```python
from build123d import *

# Parameters (mm, degrees)
F0_W     = 60
F0_H     = 40
F1_DEPTH = 10
F2_W     = 20
F2_H     = 40
F3_DEPTH = 20
F4_W     = 20
F4_H     = 10.2027570456
F5_DEPTH = 10
F6_DEPTH = 10


with BuildPart() as f1:
    # F0 (on Top) → F1 (new body)
    with BuildSketch(Plane.XY):
        with Locations((30, 20)):
            Rectangle(F0_W, F0_H)
    extrude(amount=F1_DEPTH)

    # F2 (on face) → F3 (join)
    with BuildSketch(Plane.XY.offset(10)):
        with Locations((10, 20)):
            Rectangle(F2_W, F2_H)
    extrude(amount=F3_DEPTH)

    # F4 (on face) → F5 (join)
    with BuildSketch(Plane.XY.offset(10)):
        with Locations((30, 34.8986214772)):
            Rectangle(F4_W, F4_H)
        with Locations((30, 5.1013785228)):
            Rectangle(F4_W, F4_H)
    extrude(amount=F5_DEPTH)

    # F4 (on face) → F6 (join)
    with BuildSketch(Plane.XY.offset(10)):
        with Locations((30, 34.8986214772)):
            Rectangle(F4_W, F4_H)
    extrude(amount=F6_DEPTH)


solid = f1.part
```
The model under review builds one solid part; all positions refer to its coordinate system, in mm. A direction names the side the tool comes from. Round coordinates to 2 decimals unless told otherwise and drop trailing zeros. Order: outer loops, then holes, each group sorted by start corner. A loop starts at its lowest first (then second) coordinate and runs counter-clockwise, first axis right, second up. Notation, with made-up numbers: (-21.75, -24) -> (5.25, -24) arc R16 cw to (5.25, -10) -> close; hole circle Ø5 at (50, -28.5). An arc over 180 degrees is marked (long way). One line per item, written item: value. Start each with the question number.
Q1. Take a section at B-B (z = 14.25). Write out the cut boundary in (x, y), and give its area (3 significant figures).
Q2. Wall thickness on line 1 (Y direction, x = 32, z = 19); line 2 (Z direction, x = 44, y = 3.5); line 3 (X direction, y = 29.5, z = 21.25): over which ranges is each line inside the solid? List them lowest first.
Q3. Take a section at A-A (x = 23). Write out the cut boundary in (y, z), and give its area (3 significant figures).
Q4. Machinability: for faces 1 (the face through (40, 35, 15)), 2 (the face through (30, 29.797, 15)), 3 (the face through (30, 20, 0)), which of the approach directions +Z, -Z, +X, -X, +Y, -Y give a long, thin tool a straight path to every point of the face, cutting with its end or side? Answer none if there is none.
Q5. Clearance check with flat-ended pins moving along their axes: pin 1 Ø11 at (y, z) = (7, 13.5) entering from +X; pin 2 Ø5 at (y, z) = (35.5, 15.5) entering from +X; pin 3 Ø5 at (x, y) = (33, 3.5) entering from +Z; pin 4 Ø6 at (y, z) = (10, 24) entering from +X. State where each tip first meets the part, or that it passes through.
Q6. Take a section at C-C (y = 17.5). Write out the cut boundary in (x, z), and give its area (3 significant figures).
Q7. Take a section at D-D (x = 44.5). Write out the cut boundary in (y, z), and give its area (3 significant figures).
Reported:
1. outline: (0, 0) -> (40, 0) -> (40, 10.2) -> (20, 10.2) -> (20, 29.8) -> (40, 29.8) -> (40, 40) -> (0, 40) -> close
1. area: 1,210 mm2
2. line 1: y = 0 to 10.2, 29.8 to 40
2. line 2: z = 0 to 10
2. line 3: x = 0 to 20
3. outline: (0, 0) -> (40, 0) -> (40, 20) -> (29.8, 20) -> (29.8, 10) -> (10.2, 10) -> (10.2, 20) -> (0, 20) -> close
3. area: 604 mm2
4. face 1: +Z, +X, +Y, -Y
4. face 2: +Z, +X
4. face 3: -Z, +X, -X, +Y, -Y
5. pin 1: stops at x = 60
5. pin 2: stops at x = 40
5. pin 3: stops at z = 20
5. pin 4: stops at x = 20
6. outline: (0, 0) -> (60, 0) -> (60, 10) -> (20, 10) -> (20, 30) -> (0, 30) -> close
6. area: 1,000 mm2
7. outline: (0, 0) -> (40, 0) -> (40, 10) -> (0, 10) -> close
7. area: 400 mm2
